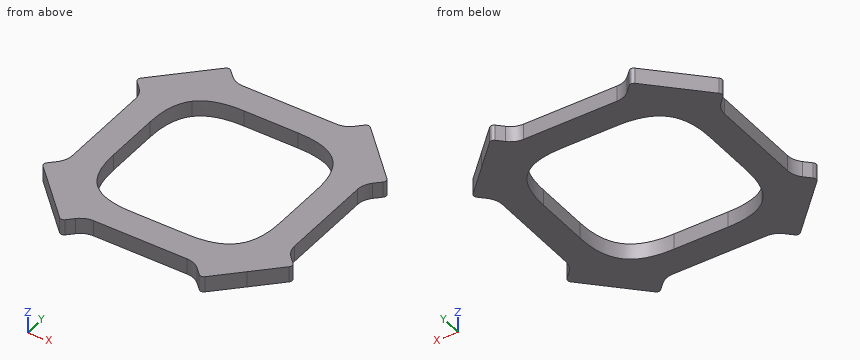
```python
from build123d import *

# Parameters (mm, degrees)
F1_DEPTH = 4


# Not quite as in the source:
# - a feature names something its author has since deleted; it is built from what else it names


with BuildPart() as f1:
    # F0 (on Top) → F1 (new body)
    with BuildSketch(Plane.XY):
        Polygon((-108.5178543984, -51.6479864335), (-108.5178543984, -37.9322576809), (-115.5178543984, -30.9322576809), (-115.5178543984, -33.0033254928), (-115.5178543984, -56.5769186216), (-115.5178543984, -58.6479864335), align=None)
        with BuildLine():
            Line((-115.5178543984, -33.0033254928), (-115.5178543984, -30.9322576809))
            Line((-115.5178543984, -30.9322576809), (-116.982320508, -29.4677915713))
            ThreePointArc((-116.982320508, -29.4677915713), (-115.89845674, -31.0899083208), (-115.5178543984, -33.0033254928))
        make_face()
        with BuildLine():
            Line((-58.0533882883, -29.4677915708), (-59.5178543984, -30.9322576809))
            Line((-59.5178543984, -30.9322576809), (-59.5178543984, -33.0033254928))
            ThreePointArc((-59.5178543984, -33.0033254928), (-59.1372520566, -31.0899083205), (-58.0533882883, -29.4677915708))
        make_face()
        Polygon((-66.5178543984, -37.9322576809), (-66.5178543984, -51.6479864335), (-59.5178543984, -58.6479864335), (-59.5178543984, -56.5769186216), (-59.5178543984, -33.0033254928), (-59.5178543984, -30.9322576809), align=None)
        with BuildLine():
            Line((-59.5178543984, -56.5769186216), (-59.5178543984, -58.6479864335))
            Line((-59.5178543984, -58.6479864335), (-58.0533883237, -60.1124525081))
            ThreePointArc((-58.0533883237, -60.1124525081), (-59.1372520662, -58.4903357707), (-59.5178543984, -56.5769186216))
        make_face()
        with BuildLine():
            Line((-116.982320508, -60.1124525431), (-115.5178543984, -58.6479864335))
            Line((-115.5178543984, -58.6479864335), (-115.5178543984, -56.5769186216))
            ThreePointArc((-115.5178543984, -56.5769186216), (-115.89845674, -58.4903357936), (-116.982320508, -60.1124525431))
        make_face()
        Polygon((-101.3757187746, -16.7901220572), (-94.3757187746, -23.7901220572), (-80.6599900221, -23.7901220572), (-73.6599900221, -16.7901220572), (-75.731057834, -16.7901220572), (-99.3046509628, -16.7901220572), align=None)
        with BuildLine():
            Line((-102.8401848842, -15.3256559476), (-101.3757187746, -16.7901220572))
            Line((-101.3757187746, -16.7901220572), (-99.3046509628, -16.7901220572))
            ThreePointArc((-99.3046509628, -16.7901220572), (-101.2180681347, -16.4095197156), (-102.8401848842, -15.3256559476))
        make_face()
        with BuildLine():
            Line((-75.731057834, -16.7901220572), (-73.6599900221, -16.7901220572))
            Line((-73.6599900221, -16.7901220572), (-72.1955238561, -15.3256558912))
            ThreePointArc((-72.1955238561, -15.3256558912), (-73.8176406251, -16.4095197003), (-75.731057834, -16.7901220572))
        make_face()
        Polygon((-73.6599900221, -72.7901220572), (-80.6599900221, -65.7901220572), (-94.3757187746, -65.7901220572), (-101.3757187746, -72.7901220572), (-99.3046509628, -72.7901220572), (-75.731057834, -72.7901220572), align=None)
        with BuildLine():
            Line((-99.3046509628, -72.7901220572), (-101.3757187746, -72.7901220572))
            Line((-101.3757187746, -72.7901220572), (-102.8401848842, -74.2545881668))
            ThreePointArc((-102.8401848842, -74.2545881668), (-101.2180681347, -73.1707243988), (-99.3046509628, -72.7901220572))
        make_face()
        with BuildLine():
            Line((-72.1955239691, -74.2545881102), (-73.6599900221, -72.7901220572))
            Line((-73.6599900221, -72.7901220572), (-75.731057834, -72.7901220572))
            ThreePointArc((-75.731057834, -72.7901220572), (-73.8176406989, -73.1707243835), (-72.1955239691, -74.2545881102))
        make_face()
        with BuildLine():
            Line((-105.1967865865, -27.1111898691), (-112.1958810618, -20.1120953938))
            Line((-112.1958810618, -20.1120953938), (-118.5598420925, -26.4760564245))
            ThreePointArc((-118.5598420925, -26.4760564245), (-118.8527353113, -27.1831632057), (-118.5598420925, -27.8902699868))
            Line((-118.5598420925, -27.8902699868), (-116.982320508, -29.4677915713))
            Line((-116.982320508, -29.4677915713), (-115.5178543984, -30.9322576809))
            Line((-115.5178543984, -30.9322576809), (-108.5178543984, -37.9322576809))
            add(Edge.make_bspline(
                [(-108.5178543984, -37.9322576809), (-108.5178543984, -32.9322576809), (-107.4823204924, -29.396723775), (-105.1967865865, -27.1111898691)],
                knots=[0, 0, 0, 0, 10, 10, 10, 10], degree=3))
        make_face()
        with BuildLine():
            Line((-105.8319200311, -13.7481343631), (-112.1958810618, -20.1120953938))
            Line((-112.1958810618, -20.1120953938), (-105.1967865865, -27.1111898691))
            add(Edge.make_bspline(
                [(-105.1967865865, -27.1111898691), (-102.9112526806, -24.8256559631), (-99.3757187746, -23.7901220572), (-94.3757187746, -23.7901220572)],
                knots=[10, 10, 10, 10, 20, 20, 20, 20], degree=3))
            Line((-94.3757187746, -23.7901220572), (-101.3757187746, -16.7901220572))
            Line((-101.3757187746, -16.7901220572), (-102.8401848842, -15.3256559476))
            Line((-102.8401848842, -15.3256559476), (-104.4177064687, -13.7481343631))
            ThreePointArc((-104.4177064687, -13.7481343631), (-105.1248132499, -13.4552411443), (-105.8319200311, -13.7481343631))
        make_face()
        with BuildLine():
            Line((-73.6599900221, -16.7901220572), (-80.6599900221, -23.7901220572))
            add(Edge.make_bspline(
                [(-80.6599900221, -23.7901220572), (-75.6599900221, -23.7901220572), (-72.1244561162, -24.8256559631), (-69.8389222102, -27.1111898691)],
                knots=[0, 0, 0, 0, 10, 10, 10, 10], degree=3))
            Line((-69.8389222102, -27.1111898691), (-62.839827735, -20.1120953938))
            Line((-62.839827735, -20.1120953938), (-69.2037887656, -13.7481343631))
            ThreePointArc((-69.2037887656, -13.7481343631), (-69.9108955468, -13.4552411443), (-70.618002328, -13.7481343631))
            Line((-70.618002328, -13.7481343631), (-72.1955238561, -15.3256558912))
            Line((-72.1955238561, -15.3256558912), (-73.6599900221, -16.7901220572))
        make_face()
        with BuildLine():
            Line((-62.839827735, -20.1120953938), (-69.8389222102, -27.1111898691))
            add(Edge.make_bspline(
                [(-69.8389222102, -27.1111898691), (-67.5533883043, -29.396723775), (-66.5178543984, -32.9322576809), (-66.5178543984, -37.9322576809)],
                knots=[10, 10, 10, 10, 20, 20, 20, 20], degree=3))
            Line((-66.5178543984, -37.9322576809), (-59.5178543984, -30.9322576809))
            Line((-59.5178543984, -30.9322576809), (-58.0533882883, -29.4677915708))
            Line((-58.0533882883, -29.4677915708), (-56.4758667043, -27.8902699868))
            ThreePointArc((-56.4758667043, -27.8902699868), (-56.1829734855, -27.1831632057), (-56.4758667043, -26.4760564245))
            Line((-56.4758667043, -26.4760564245), (-62.839827735, -20.1120953938))
        make_face()
        with BuildLine():
            add(Edge.make_bspline(
                [(-69.8389222102, -62.4690542453), (-67.5533883043, -60.1835203394), (-66.5178543984, -56.6479864335), (-66.5178543984, -51.6479864335)],
                knots=[10, 10, 10, 10, 20, 20, 20, 20], degree=3))
            Line((-69.8389222102, -62.4690542453), (-62.839827735, -69.4681487206))
            Line((-62.839827735, -69.4681487206), (-56.4758667043, -63.1041876899))
            ThreePointArc((-56.4758667043, -63.1041876899), (-56.1829734855, -62.3970809087), (-56.4758667043, -61.6899741276))
            Line((-56.4758667043, -61.6899741276), (-58.0533883237, -60.1124525081))
            Line((-58.0533883237, -60.1124525081), (-59.5178543984, -58.6479864335))
            Line((-59.5178543984, -58.6479864335), (-66.5178543984, -51.6479864335))
        make_face()
        with BuildLine():
            Line((-62.839827735, -69.4681487206), (-69.8389222102, -62.4690542453))
            add(Edge.make_bspline(
                [(-80.6599900221, -65.7901220572), (-75.6599900221, -65.7901220572), (-72.1244561162, -64.7545881513), (-69.8389222102, -62.4690542453)],
                knots=[0, 0, 0, 0, 10, 10, 10, 10], degree=3))
            Line((-80.6599900221, -65.7901220572), (-73.6599900221, -72.7901220572))
            Line((-73.6599900221, -72.7901220572), (-72.1955239691, -74.2545881102))
            Line((-72.1955239691, -74.2545881102), (-70.618002328, -75.8321097513))
            ThreePointArc((-70.618002328, -75.8321097513), (-69.9108955468, -76.1250029701), (-69.2037887656, -75.8321097513))
            Line((-69.2037887656, -75.8321097513), (-62.839827735, -69.4681487206))
        make_face()
        with BuildLine():
            add(Edge.make_bspline(
                [(-105.1967865865, -62.4690542453), (-102.9112526806, -64.7545881513), (-99.3757187746, -65.7901220572), (-94.3757187746, -65.7901220572)],
                knots=[10, 10, 10, 10, 20, 20, 20, 20], degree=3))
            Line((-105.1967865865, -62.4690542453), (-112.1958810618, -69.4681487206))
            Line((-112.1958810618, -69.4681487206), (-105.8319200311, -75.8321097513))
            ThreePointArc((-105.8319200311, -75.8321097513), (-105.1248132499, -76.1250029701), (-104.4177064687, -75.8321097513))
            Line((-104.4177064687, -75.8321097513), (-102.8401848842, -74.2545881668))
            Line((-102.8401848842, -74.2545881668), (-101.3757187746, -72.7901220572))
            Line((-101.3757187746, -72.7901220572), (-94.3757187746, -65.7901220572))
        make_face()
        with BuildLine():
            add(Edge.make_bspline(
                [(-108.5178543984, -51.6479864335), (-108.5178543984, -56.6479864335), (-107.4823204924, -60.1835203394), (-105.1967865865, -62.4690542453)],
                knots=[0, 0, 0, 0, 10, 10, 10, 10], degree=3))
            Line((-108.5178543984, -51.6479864335), (-115.5178543984, -58.6479864335))
            Line((-115.5178543984, -58.6479864335), (-116.982320508, -60.1124525431))
            Line((-116.982320508, -60.1124525431), (-118.5598420925, -61.6899741276))
            ThreePointArc((-118.5598420925, -61.6899741276), (-118.8527353113, -62.3970809087), (-118.5598420925, -63.1041876899))
            Line((-118.5598420925, -63.1041876899), (-112.1958810618, -69.4681487206))
            Line((-112.1958810618, -69.4681487206), (-105.1967865865, -62.4690542453))
        make_face()
    extrude(amount=F1_DEPTH)


solid = f1.part
```
Check sheet for the modelled part. Datum: model origin and axes. Units: mm. Give positions to 0.01 mm unless a question says otherwise; leave off trailing zeros. Order: outer loops, then holes, each group sorted by start corner. A loop starts at its lowest first (then second) coordinate and runs counter-clockwise, first axis right, second up. Notation, with made-up numbers: M 53,-29 L 93,-29 A12 cw 93,-19 Z; hole C -14.75,19.25 d9. An arc over 180 degrees is marked long. Answer in a Markdown table with one row per item. Add a question column.
Q1. Thickness scan on L1, parallel to Y at x = -95, z = 2.7; L2, parallel to X at y = -41, z = 3.2; L3, parallel to Y at x = -75.5, z = 3.35. Record the ranges inside material, lowest first.
Q2. Gauge pin test, flat ends, axial feed: pin 1 Ø8 at (x, y) = (-103, -58) entering from +Z; pin 2 Ø2 at (y, z) = (-50.5, 1.5) entering from -X; pin 3 Ø2 at (x, z) = (-77.5, 3.5) entering from -Y; pin 4 Ø2 at (y, z) = (-47.5, 1.5) entering from +X. Record the tip position at first contact, or that the pin passes through.
Q3. Sectioned sample at A-A, the plane y = -42.5. Record the boundary of the cut face in (x, z), and give its area (3 significant figures).
Q4. Sectioned sample at B-B, the plane x = -111.5. Record the boundary of the cut face in (y, z).
Q5. Sectioned sample at C-C, the plane y = -18. Record the boundary of the cut face in (x, z).
Verdict:
| question | item | result |
|---|---|---|
| 1 | L1 | -72.79 to -65.78, -23.8 to -16.79 |
| 1 | L2 | -115.52 to -108.52, -66.52 to -59.52 |
| 1 | L3 | -72.8 to -65.31, -24.27 to -16.78 |
| 2 | pin 1 | through |
| 2 | pin 2 | x = -115.52 |
| 2 | pin 3 | y = -72.79 |
| 2 | pin 4 | x = -59.52 |
| 3 | outline | M -115.52,0 L -108.52,0 L -108.52,4 L -115.52,4 Z; M -66.52,0 L -59.52,0 L -59.52,4 L -66.52,4 Z |
| 3 | area | 56.0 mm² |
| 4 | outline | M -70.16,0 L -19.42,0 L -19.42,4 L -70.16,4 Z |
| 5 | outline | M -110.08,0 L -64.95,0 L -64.95,4 L -110.08,4 Z |
